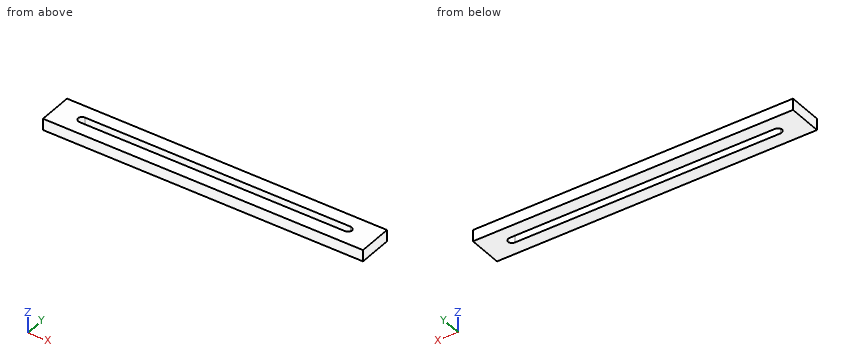
```python
from build123d import *

# Parameters (mm, degrees)
F0_W        = 140
F0_H        = 15
F0_W_2      = 120
F0_H_2      = 3.4
F1_DEPTH    = 5
F2_T1_DEPTH = 5


# Not quite as in the source:
# - a fillet or chamfer that OpenCascade refuses, or shapes differently, is made with other operations: its cross-section is extruded or revolved along the edge and cut away or added


with BuildPart() as f1:
    # F0 (on Top) → F1 (new body)
    with BuildSketch(Plane.XY):
        Rectangle(F0_W, F0_H)
        Rectangle(F0_W_2, F0_H_2, mode=Mode.SUBTRACT)
    extrude(amount=F1_DEPTH)

    # F2: fillet of radius 2 on 4 edges, made by hand

    # F2_s2 → F2_t1 (join)
    with BuildSketch(Plane.XY):
        with BuildLine():
            ThreePointArc((-58, 1.7), (-59.4142135624, 1.1142135624), (-60, -0.3))
            Line((-60, -0.3), (-60, 1.7))
            Line((-60, 1.7), (-58, 1.7))
        make_face()
        with BuildLine():
            ThreePointArc((-58, -1.7), (-59.4142135624, -1.1142135624), (-60, 0.3))
            Line((-60, 0.3), (-60, -1.7))
            Line((-60, -1.7), (-58, -1.7))
        make_face()
        with BuildLine():
            ThreePointArc((58, 1.7), (59.4142135624, 1.1142135624), (60, -0.3))
            Line((60, -0.3), (60, 1.7))
            Line((60, 1.7), (58, 1.7))
        make_face()
        with BuildLine():
            ThreePointArc((60, 0.3), (59.4142135624, -1.1142135624), (58, -1.7))
            Line((58, -1.7), (60, -1.7))
            Line((60, -1.7), (60, 0.3))
        make_face()
    extrude(amount=F2_T1_DEPTH)


solid = f1.part
```
CAD build for the part. Positions are in the model's coordinates, mm. Coordinates: 2 decimals unless noted, no trailing zeros. Order: outer loops, then holes, each group sorted by start corner. A loop starts at its lowest first (then second) coordinate and runs counter-clockwise, first axis right, second up. Notation, with made-up numbers: (30.25, 15) - (41.25, 15) arc R20 ccw to (41.25, 51) - close; hole circle Ø9 at (54.5, 72). An arc over 180 degrees is marked (long way). Answer in a Markdown table with one row per item.
1. Slice it at B-B, the plane z = 1.9. List the corners of the cut face in (x, y), then the cut area to 3 significant figures.
Answer:
| item | result |
|---|---|
| outline | (-70, -7.5) - (70, -7.5) - (70, 7.5) - (-70, 7.5) - close; hole (-59.98, 0) arc R2 ccw to (-58, -1.7) - (58, -1.7) arc R2 ccw to (59.98, 0) arc R2 ccw to (58, 1.7) - (-58, 1.7) arc R2 ccw to start |
| area | 1,700 mm² |
2. Slice it at A-A, the plane x = -44. List the corners of the cut face in (y, z), then the cut area to 3 significant figures.
Answer:
| item | result |
|---|---|
| outline | (-7.5, 0) - (-1.7, 0) - (-1.7, 5) - (-7.5, 5) - close; (1.7, 0) - (7.5, 0) - (7.5, 5) - (1.7, 5) - close |
| area | 58.0 mm² |
3. Flat gauge pin, fed straight in: P1, Ø4, axis at x = 23.5, y = 4, coming from the -Z side. Where does the tip first touch, or does it go through?
Answer:
| item | result |
|---|---|
| P1 | z = 0 |
4. Drill centre lines: L1, parallel to Y at x = -57.5, z = 2.9; L2, parallel to X at y = 0.25, z = 0.6; L3, parallel to X at y = -1, z = 2.4. Where is each one in solid material? Low to high. Write a range as from..to.
Answer:
| item | result |
|---|---|
| L1 | -7.5..-1.7, 1.7..7.5 |
| L2 | -70..-59.92, 59.92..70 |
| L3 | -70..-59.52, 59.52..70 |
